Read the model definition and answer for the solid it produces. Units are mm, in the model's axes. Give positions to 0.01 mm unless a question says otherwise; leave off trailing zeros. Order: outer loops, then holes, each group sorted by start corner. A loop starts at its lowest first (then second) coordinate and runs counter-clockwise, first axis right, second up. Notation, with made-up numbers: (67, -2) - (86, -2) arc R8 ccw to (86, 5) - close; hole circle Ø3 at (-37, 80). An arc over 180 degrees is marked (long way). One line per item, written item: value. Start each with the question number.
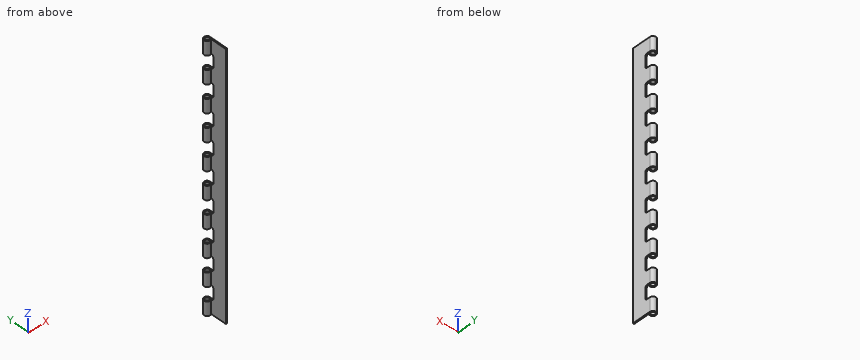
Autodesk Inventor part; units mm, degrees
ref_plane "YZ Plane" through (0, 0, 0) normal (1, 0, 0) x (0, 1, 0)
ref_plane "XZ Plane" through (0, 0, 0) normal (0, 1, 0) x (-1, 0, 0)
ref_plane "XY Plane" through (0, 0, 0) normal (0, 0, 1) x (1, 0, 0)
sketch "Sketch1" plane through (0, 0, 0) normal (0, 0, 1) x (1, 0, 0)
  line L0 (-3.3994, 19.4704) -> (-3.3994, -14.4081)
  line L1 (-3.3994, -14.4081) -> (-5.6854, -14.4081)
  arc A0 (-3.3994, 19.4704) -> (-6.6643, 14.3475) centre (-9.0509, 19.4704) ccw
  arc A1 (-5.6854, 19.4704) -> (-7.7383, 16.3714) centre (-9.0509, 19.4704) ccw
  line L2 (-7.7383, 16.3714) -> (-6.6643, 14.3475)
  line L3 (-5.6854, -14.4081) -> (-5.6854, 19.4704)
  dimension "d0" = 11.303
  dimension "d2" = 2.286
extrude "Extrusion1" add sketch "Sketch1" along normal blind 482.6
sketch "Sketch2" plane through (-3.3994, -14.4081, 0) normal (1, 0, 0) x (0, 0, -1)
  line L0 (-482.6, 33.8785) -> (-482.6, 0)
  line L1 (-457.2, 50.4757) -> (-431.8, 50.4757)
  line L2 (-431.8, 50.4757) -> (-431.8, 25.052)
  line L3 (-431.8, 25.052) -> (-457.2, 25.052)
  line L4 (-457.2, 25.052) -> (-457.2, 50.4757)
  line L5 (-482.6, 37.244) -> (0, 37.244)
  line L6 (-482.6, 33.8785) -> (-482.6, 30.7795)
  line L7 (0, 30.7795) -> (-482.6, 30.7795)
  line L8 (0, 30.7795) -> (0, 33.8785)
  line L9 (0, 33.8785) -> (-482.6, 33.8785)
  line L10 (0, 28.227) -> (-482.6, 28.227)
  dimension "d5" = 25.4
  dimension "d6" = 25.4
  dimension "d7" = 3.175
extrude "Extrusion2" cut sketch "Sketch2" against normal through all contours L9 L2 L7 L4 | L4 L5 L2 L9 | L7 L2 L10 L4 | L4 L1 L2 L5 | L10 L2 L3 L4
fillet "Fillet1" radius 3.175 2 edges at (-4.5424, 10.6439, 431.8) (-4.5424, 10.6439, 457.2)
pattern_linear "Rectangular Pattern1" count 9 spacing 50.8 along (0, 0, -1) of "Extrusion2", "Fillet1"
properties part number "FE-00004-03A"
1) Find the intervals of material crossed by probe 1 along X at (y, z) = (20, 20.5); probe 2 along X at (y, z) = (-12.5, 105); probe 3 along X at (y, z) = (22.5, 165.5), in increasing order. Write a range as from..to.
2) Section C-C on z = 345.5 is taken. Write down the section's boundary in (x, y).
3) Section A-A on z = 265 is taken. Write down the section's boundary in (x, y).
4) Section B-B on y = 0 is taken. Write down the section's boundary in (x, z).
5) Each of these flat-tipped pins is pushed along its axis until it touches: pin 1 (2.5 mm diameter, centred on x = -5, z = 87.5, fed in from +Y); pin 2 (4 mm diameter, centred on y = -8, z = 118, fed in from -X). Where does it stop, or does it pass through?
Solved:
1. probe 1: x = -14.68..-12.37, -5.73..-3.42
1. probe 2: x = -5.69..-3.4
1. probe 3: x = -13.82..-10.52, -7.59..-4.28
2. outline: (-5.69, -14.41) - (-3.4, -14.41) - (-3.4, 10.64) - (-5.69, 10.64) - close
3. outline: (-7.74, 16.37) arc R3.37 cw (long way) to (-5.69, 19.47) - (-5.69, -14.41) - (-3.4, -14.41) - (-3.4, 19.47) arc R5.65 ccw (long way) to (-6.66, 14.35) - close
4. outline: (-5.69, 0) - (-3.4, 0) - (-3.4, 482.6) - (-5.69, 482.6) - close
5. pin 1: stops at y = 10.64
5. pin 2: stops at x = -5.69
